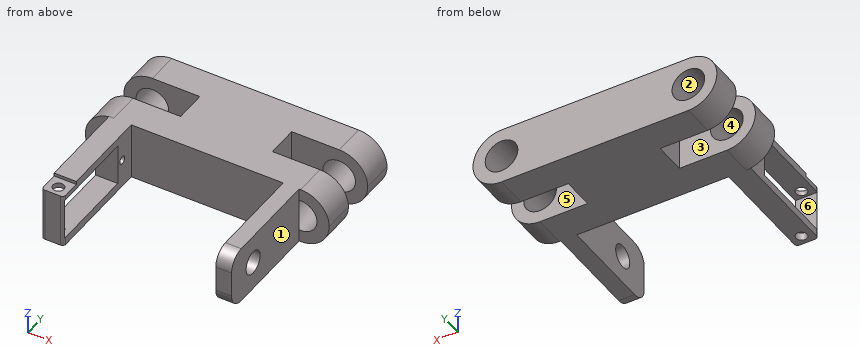
from build123d import *

# Parameters (mm, degrees)
F0_R         = 5.15
F1_DEPTH     = 30
F2_W         = 26.2453191746
F2_H         = 10
F2_W_2       = 30.2312795687
F3_DEPTH     = 25
F4_W         = 5
F4_H         = 18
F4_W_2       = 7
F5_DEPTH     = 35
F6_W         = 27.5
F6_H         = 13
F6_R         = 1.25
F7_DEPTH     = 25
F8_R         = 3.65
F9_DEPTH     = 25
F10_R        = 5
F11_R        = 1.75
F12_DEPTH    = 25
F13_W        = 7
F13_H        = 6.5
F14_DEPTH    = 1
F15_T1_DEPTH = 22


# Not quite as in the source:
# - a fillet or chamfer that OpenCascade refuses, or shapes differently, is made with other operations: its cross-section is extruded or revolved along the edge and cut away or added


with BuildPart() as f1:
    # F0 (on Front) → F1 (new body)
    with BuildSketch(Plane.XZ):
        with BuildLine():
            ThreePointArc((-59, -9), (-52.6360389693, -6.3639610307), (-50, 0))
            ThreePointArc((-50, 0), (-52.6360389693, 6.3639610307), (-59, 9))
            ThreePointArc((-59, 9), (-68, 0), (-59, -9))
        make_face()
        with Locations((-59, 0)):
            Circle(F0_R, mode=Mode.SUBTRACT)
        with BuildLine():
            ThreePointArc((-59, 9), (-52.6360389693, 6.3639610307), (-50, 0))
            ThreePointArc((-50, 0), (-52.6360389693, -6.3639610307), (-59, -9))
            Line((-59, -9), (0, -9))
            ThreePointArc((0, -9), (-9, 0), (0, 9))
            Line((0, 9), (-59, 9))
        make_face()
        with BuildLine():
            ThreePointArc((9, 0), (6.3639610307, 6.3639610307), (0, 9))
            ThreePointArc((0, 9), (-9, 0), (0, -9))
            ThreePointArc((0, -9), (6.3639610307, -6.3639610307), (9, 0))
        make_face()
        Circle(F0_R, mode=Mode.SUBTRACT)
    extrude(amount=F1_DEPTH)

    # F2 (on face) → F3 (cut)
    with BuildSketch(Plane.XY.offset(9)):
        with Locations((-1.8773404127, -15)):
            Rectangle(F2_W, F2_H)
        with Locations((-59.1156397844, -15)):
            Rectangle(F2_W_2, F2_H)
    extrude(amount=-F3_DEPTH, mode=Mode.SUBTRACT)

    # F4 (on face) → F5 (join)
    with BuildSketch(Plane.XZ.offset(30)):
        with Locations((-3, 0)):
            Rectangle(F4_W, F4_H)
        with Locations((-57, 0)):
            Rectangle(F4_W_2, F4_H)
    extrude(amount=F5_DEPTH)

    # F6 (on face) → F7 (cut)
    with BuildSketch(Plane(origin=(-60.5, 0, 0), x_dir=(0, -1, 0), z_dir=(-1, 0, 0))):
        with Locations((50.75, 0)):
            Rectangle(F6_W, F6_H)
        with Locations((34.7, 0)):
            Circle(F6_R)
    extrude(amount=-F7_DEPTH, mode=Mode.SUBTRACT)

    # F8 (on face) → F9 (cut)
    with BuildSketch(Plane(origin=(-5.5, 0, 0), x_dir=(0, -1, 0), z_dir=(-1, 0, 0))):
        with Locations((53.85, 0)):
            Circle(F8_R)
    extrude(amount=-F9_DEPTH, mode=Mode.SUBTRACT)

    # F10
    f10_edges = [f1.edges().sort_by_distance(p)[0] for p in [
        (-3, -65, 9),
        (-3, -65, -9),
    ]]
    fillet(f10_edges, radius=F10_R)

    # F11 (on face) → F12 (cut)
    with BuildSketch(Plane.XY.offset(9)):
        with Locations((-57, -62)):
            Circle(F11_R)
    extrude(amount=-F12_DEPTH, mode=Mode.SUBTRACT)

    # F13 (on face) → F14 (cut)
    with BuildSketch(Plane.XY.offset(9)):
        with Locations((-57, -61.75)):
            Rectangle(F13_W, F13_H)
    extrude(amount=-F14_DEPTH, mode=Mode.SUBTRACT)

    # F15: fillet of radius 1 on 2 edges, made by hand

    # F15_s2 → F15_t1 (cut)
    with BuildSketch(Plane.XY.offset(-11.5)):
        with BuildLine():
            ThreePointArc((-59.5, -65), (-60.2071067812, -64.7071067812), (-60.5, -64))
            Line((-60.5, -64), (-60.5, -65))
            Line((-60.5, -65), (-59.5, -65))
        make_face()
        with BuildLine():
            ThreePointArc((-53.5, -64), (-53.7928932188, -64.7071067812), (-54.5, -65))
            Line((-54.5, -65), (-53.5, -65))
            Line((-53.5, -65), (-53.5, -64))
        make_face()
    extrude(amount=F15_T1_DEPTH, mode=Mode.SUBTRACT)


solid = f1.part
Here's how the part is built. I have some questions about the finished solid (model axes, mm). Face numbers are marked on the shaded views. A direction names the side the tool comes from. Give positions to 0.01 mm unless a question says otherwise; leave off trailing zeros. Write each loop counter-clockwise with the first axis right and the second up, starting at its lowest first coordinate (ties: lowest second). Pieces come first, ordered by that corner, then holes. Notation, with made-up numbers: (83.25, -29.75) -> (137.25, -29.75) arc R31 ccw to (137.25, 9.25) -> close; hole circle Ø3 at (64, -36.5). An arc over 180 degrees is marked (long way). Use one line per item in the form item = value. Start each with the question number.
1. Will these pins go through, and if not, where does the flat tip stop? pin 1 Ø3 at (x, z) = (-1, -4.5) entering from +Y; pin 2 Ø8 at (y, z) = (-32.5, -6.5) entering from +X; pin 3 Ø8.5 at (x, z) = (-65.5, -1) entering from -Y; pin 4 Ø3.5 at (x, z) = (-56.5, -1) entering from +Y.
2. Imagine slicing it at C-C on y = -53.85. List the corners of the cut face in (x, z) for me.
3. Thinking about a two-plate mould opening in X: for the marked faces 1, 2 and 3, which applies, +X half, -X half, draft (parallel to the pull), parting line (faces both ways), or undercut?
4. On a 3-axis mill with a long thin cutter (end or side, diameter ignored), from which of +Z, -Z, +X, -X, +Y, -Y can I reach the whole of each face in a straight line? I mean the marked faces 4, 5 and 6. Say none if no direction works.
5. Imagine slicing it at D-D on y = -8. List the corners of the cut face in (x, z) for me.
6. If I drill on L1, parallel to Y at x = -57, z = 7.15; L2, parallel to Y at x = -56, z = 3.5; L3, parallel to X at y = -60, z = 7.5, over which ranges is the centre line in solid material (lowest first)?
7. Imagine slicing it at A-A on y = -45. List the corners of the cut face in (x, z) for me, plus the area to 3 significant figures.
8. Imagine slicing it at B-B on x = -52.5. List the corners of the cut face in (y, z) for me.
Entries:
q1.pin_1 = 0
q1.pin_2 = 8.34
q1.pin_3 = -30
q1.pin_4 = -30
q2.outline = (-60.5, -9) -> (-53.5, -9) -> (-53.5, -6.5) -> (-60.5, -6.5) -> close; (-60.5, 6.5) -> (-53.5, 6.5) -> (-53.5, 9) -> (-60.5, 9) -> close; (-5.5, -9) -> (-0.5, -9) -> (-0.5, -3.65) -> (-5.5, -3.65) -> close; (-5.5, 3.65) -> (-0.5, 3.65) -> (-0.5, 9) -> (-5.5, 9) -> close
q3.face_1 = +X half
q3.face_2 = undercut
q3.face_3 = draft
q4.face_4 = +Y
q4.face_5 = +Z, -Z, +X
q4.face_6 = -X
q5.outline = (-59, -9) -> (0, -9) arc R9 ccw to (0, 9) -> (-59, 9) arc R9 ccw to start; hole circle Ø10.3 at (-59, 0); hole circle Ø10.3 at (0, 0)
q6.L1 = -65 to -63.75, -60.25 to -20, -10 to 0
q6.L2 = -65 to -64.5, -37 to -30
q6.L3 = -60.5 to -53.5, -5.5 to -0.5
q7.outline = (-60.5, -9) -> (-53.5, -9) -> (-53.5, -6.5) -> (-60.5, -6.5) -> close; (-60.5, 6.5) -> (-53.5, 6.5) -> (-53.5, 9) -> (-60.5, 9) -> close; (-5.5, -9) -> (-0.5, -9) -> (-0.5, 9) -> (-5.5, 9) -> close
q7.area = 125 mm²
q8.outline = (-30, -9) -> (-20, -9) -> (-20, 9) -> (-30, 9) -> close; (-10, -9) -> (0, -9) -> (0, 9) -> (-10, 9) -> close
